Check sheet for the drawn part. Datum: minimum x, y, z corner. Units: mm. A direction names the side the tool comes from. Round coordinates to 2 decimals unless told otherwise and drop trailing zeros. Order: outer loops, then holes, each group sorted by start corner. A loop starts at its lowest first (then second) coordinate and runs counter-clockwise, first axis right, second up.
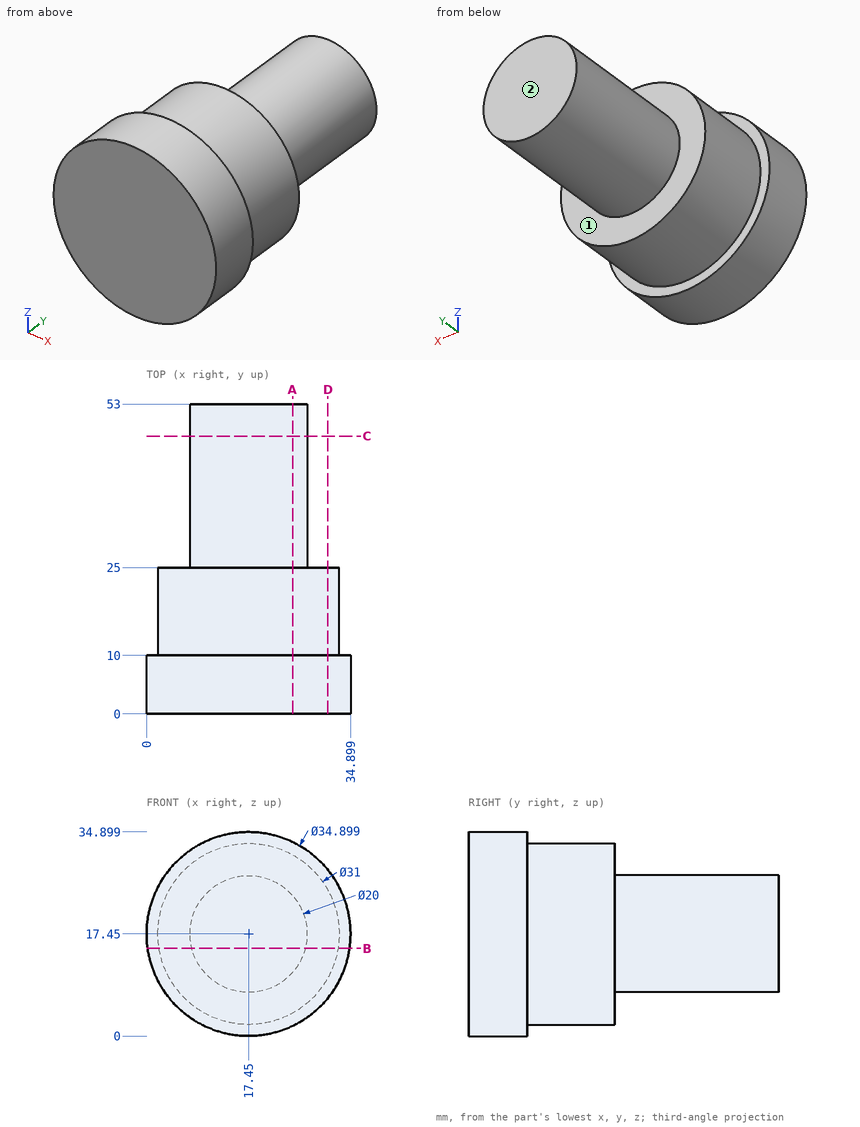
(1) Sectioned sample at A-A, the plane x = 25. Record the cut outline in (y, z), and give its area (3 significant figures).
Returned:
outline: (0, 1.72) - (10, 1.72) - (10, 3.91) - (25, 3.91) - (25, 10.89) - (53, 10.89) - (53, 24.01) - (25, 24.01) - (25, 30.99) - (10, 30.99) - (10, 33.18) - (0, 33.18) - close
area: 1,090 mm2
(2) Depth check by flat-ended pin: P1, Ø4, axis at x = 20.5, y = 46.5, coming from the -Z side (1 decimal); P2, Ø6, axis at y = 37, z = 28.5, coming from the -X side (1 decimal); P3, Ø6, axis at x = 10, y = 35, coming from the -Z side (1 decimal). Enter the tip coordinate at first touch or a pass-through.
Returned:
P1: stops at z = 7.5
P2: stops at x = 11.5
P3: stops at z = 8.5
(3) Material ranges on line 1 (Y direction, x = 24, z = 27.5); line 2 (X direction, y = 27.5, z = 17.5); line 3 (Y direction, x = 24, z = 33), recorded low to high.
Returned:
line 1: y = 0 to 25
line 2: x = 7.45 to 27.45
line 3: y = 0 to 10
(4) Sectioned sample at D-D, the plane x = 31. Record the cut outline in (y, z) (1 decimal).
Returned:
outline: (0, 6.5) - (10, 6.5) - (10, 9.9) - (25, 9.9) - (25, 25) - (10, 25) - (10, 28.4) - (0, 28.4) - close
(5) Sectioned sample at B-B, the plane z = 15. Record the cut outline in (x, y) (1 decimal).
Returned:
outline: (0.2, 0) - (34.7, 0) - (34.7, 10) - (32.8, 10) - (32.8, 25) - (27.1, 25) - (27.1, 53) - (7.8, 53) - (7.8, 25) - (2.1, 25) - (2.1, 10) - (0.2, 10) - close
(6) Sectioned sample at C-C, the plane y = 47.5. Record the cut outline in (x, z).
Returned:
outline: circle Ø20 at (17.45, 17.45)
(7) Set-up check for the marked faces 1 and 2: record each of +Z, -Z, +X, -X, +Y, -Y from which the full face is reachable in a straight line by a thin tool's end or side.
Returned:
face 1: +Y
face 2: +Z, -Z, +X, -X, +Y
